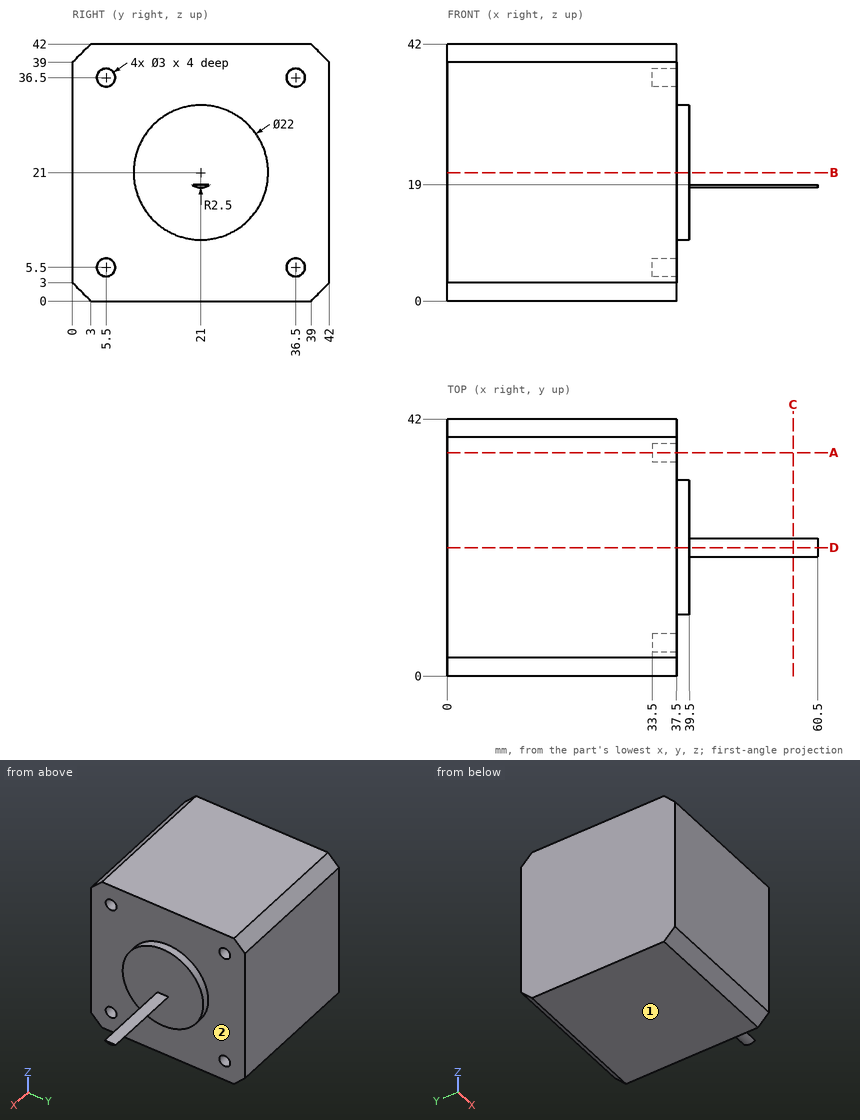
Here's the drawing with two shaded views (mm, measured from the low corner). I have some questions. A direction names the side the tool comes from. Coordinates: 2 decimals unless noted, no trailing zeros. Order: outer loops, then holes, each group sorted by start corner. A loop starts at its lowest first (then second) coordinate and runs counter-clockwise, first axis right, second up.
Item 1: For P1, Ø0.9, axis at y = 5, z = 6, coming from the +X side; P2, Ø1, axis at y = 18, z = 23, coming from the +X side; P3, Ø3.5, axis at y = 36, z = 37, coming from the +X side, each with a flat end and sliding along its axis, tell me the tip position at first contact or that it passes through.
Result sheet:
P1: stops at x = 33.5
P2: stops at x = 39.5
P3: stops at x = 37.5
Item 2: If we section it at C-C on x = 56.5: List the corners of the cut face in (y, z) for me.
Result sheet:
outline: (19.5, 19) arc R2.5 ccw to (22.5, 19) - close
Item 3: For the marked faces 1 and 2, which set-ups out of +Z, -Z, +X, -X, +Y, -Y let a thin tool reach every point of the face, with its end or its side?
Result sheet:
face 1: -Z, +X, -X, +Y, -Y
face 2: +X
Item 4: I need wall thicknesses on line 1 (Z direction, x = 34.6, y = 5.5); line 2 (X direction, y = 22, z = 7.5). Which ranges of each line are inside material? Lowest first, please.
Result sheet:
line 1: z = 0 to 4, 7 to 35, 38 to 42
line 2: x = 0 to 37.5
Item 5: If we section it at B-B on z = 21: List the corners of the cut face in (x, y) for me.
Result sheet:
outline: (0, 0) - (37.5, 0) - (37.5, 10) - (39.5, 10) - (39.5, 32) - (37.5, 32) - (37.5, 42) - (0, 42) - close
Item 6: If we section it at D-D on y = 21: List the corners of the cut face in (x, z) for me.
Result sheet:
outline: (0, 0) - (37.5, 0) - (37.5, 10) - (39.5, 10) - (39.5, 18.5) - (60.5, 18.5) - (60.5, 19) - (39.5, 19) - (39.5, 32) - (37.5, 32) - (37.5, 42) - (0, 42) - close
Item 7: If we section it at A-A on y = 36.5: List the corners of the cut face in (x, z) for me, plus the area to 3 significant figures.
Result sheet:
outline: (0, 0) - (37.5, 0) - (37.5, 4) - (33.5, 4) - (33.5, 7) - (37.5, 7) - (37.5, 35) - (33.5, 35) - (33.5, 38) - (37.5, 38) - (37.5, 42) - (0, 42) - close
area: 1,550 mm2
